The model under review builds one solid part; all positions refer to its coordinate system, in mm. Face numbers are marked on the shaded views. Coordinates: 2 decimals unless noted, no trailing zeros. Write each loop counter-clockwise with the first axis right and the second up, starting at its lowest first coordinate (ties: lowest second). Pieces come first, ordered by that corner, then holes. Notation, with made-up numbers: (-17, 44) - (38, 44) arc R13 ccw to (38, 50) - close; hole circle Ø4 at (77, 67.5). An arc over 180 degrees is marked (long way). Put each result on its own line as item: value.
from build123d import *

# Parameters (mm, degrees)
M3_CLEARANCE_HOLE1_D = 3.4


with BuildPart() as part:
    # Sketch1 → Revolve1 (revolve)
    with BuildSketch(Plane.XY, mode=Mode.PRIVATE) as revolve1_sk:
        Polygon((9, 0), (11, 0), (11, 8), (13, 8), (13, 0), (22, 0), (22, -2), (9, -2), align=None)
    revolve(revolve1_sk.sketch.rotate(Axis((0, 17.954019247, 0), (0, -1, 0)), 90), axis=Axis((0, 17.954019247, 0), (0, -1, 0)))

    # Sketch4 → Groove for BS 3673 P4 - B022M, Internal Circlip1 (revolve, cut)
    with BuildSketch(Plane(origin=(0, 17.954019247, 0), x_dir=(0, 0, 1), z_dir=(-1, 0, 0))):
        with BuildLine():
            Line((11.39, -11.954019247), (9.9, -11.954019247))
            Line((9.9, -11.954019247), (9.9, -10.854019247))
            Line((9.9, -10.854019247), (11.39, -10.854019247))
            ThreePointArc((11.39, -10.854019247), (11.467781746, -10.886237501), (11.5, -10.964019247))
            Line((11.5, -10.964019247), (11.5, -11.844019247))
            ThreePointArc((11.5, -11.844019247), (11.467781746, -11.921800993), (11.39, -11.954019247))
        make_face()
    revolve(axis=Axis((0, -32.045980753, 0), (0, 1, 0)), mode=Mode.SUBTRACT)

    # M3 Clearance Hole1 (through all)
    with Locations(Plane(origin=(0, 0, 0), x_dir=(1, 0, 0), z_dir=(0, 1, 0))):
        with Locations((0, 17.5), (17.5, 0), (0, -17.5), (-17.5, 0)):
            Hole(M3_CLEARANCE_HOLE1_D / 2)


solid = part.part
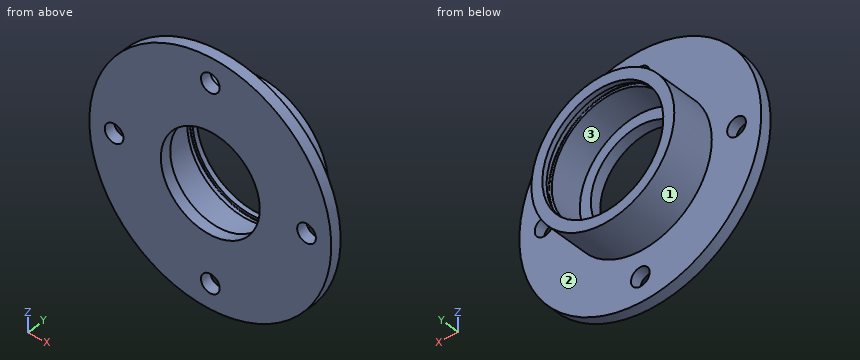
1. Consider section A-A on z = 18.5. State the section outline as (x, y) points.
Determined:
outline: (-11.91, -2) - (-1.37, -2) - (-1.37, 0) - (-11.91, 0) - close; (1.37, -2) - (11.91, -2) - (11.91, 0) - (1.37, 0) - close
2. Consider section D-D on z = 0. Give the number of separate pieces and of enclosed holes in the cut face, plus the area to 3 significant figures.
Determined:
separate pieces: 4
enclosed holes: 0
area: 69.3 mm^2
3. Consider section B-B on x = 18.5. State the section outline as (y, z) points, plus the area to 3 significant figures.
Determined:
outline: (-2, -11.91) - (0, -11.91) - (0, -1.37) - (-2, -1.37) - close; (-2, 1.37) - (0, 1.37) - (0, 11.91) - (-2, 11.91) - close
area: 42.1 mm^2
4. For pin 1 Ø4 at (y, z) = (6, -10) entering from -X; pin 2 Ø17.5 at (x, z) = (1.5, -0.5) entering from +Y; pin 3 Ø3 at (y, z) = (2.5, 10) entering from -X; pin 4 Ø2 at (x, z) = (-17.5, 0) entering from +Y, all flat-tipped, find the tip position at first contact; note any pin that passes through.
Determined:
pin 1: stops at x = -10.25
pin 2: stops at y = 0
pin 3: stops at x = -9.84
pin 4: passes through
5. To check wall thickness, follow probe 1 along X at (y, z) = (7.8, 0); probe 2 along Y at (x, z) = (8.5, 7.5); probe 3 along Y at (x, z) = (-10, 9). State the ranges of each line that lie inside material, in increasing order.
Determined:
probe 1: x = -13 to -11, 11 to 13
probe 2: y = -2 to 6, 7.1 to 8
probe 3: y = -2 to 0
6. The part is to be moulded in two halves that separate along Z. For the marked faces 1, 2 and 3, say which applies: +Z half, -Z half, draft (parallel to the pull), parting line (faces both ways), or undercut.
Determined:
face 1: parting line
face 2: draft
face 3: undercut
7. Consider section C-C on y = 4.25. State the section outline as (x, z) points, plus the area to 3 significant figures.
Determined:
outline: circle Ø26 at (0, 0); hole circle Ø22 at (0, 0)
area: 151 mm^2
